Part model, mm, in its own coordinate system. Face numbers are marked on the shaded views. A direction names the side the tool comes from. Coordinates: 2 decimals unless noted, no trailing zeros. Order: outer loops, then holes, each group sorted by start corner. A loop starts at its lowest first (then second) coordinate and runs counter-clockwise, first axis right, second up.
from build123d import *

# Parameters (mm, degrees)
F0_W     = 25.2
F0_H     = 7.2
F1_DEPTH = 58.45
F2_W     = 15.086318
F2_H     = 7.2
F3_DEPTH = 5


with BuildPart() as f1:
    # F0 (on Front) → F1 (new body, symmetric)
    with BuildSketch(Plane.XZ):
        with Locations((-28.073686, 3.6)):
            Rectangle(F0_W, F0_H)
    extrude(amount=F1_DEPTH, both=True)

    # F2 (on face) → F3 (join)
    with BuildSketch(Plane.XZ.offset(58.45)):
        with Locations((-28.144586, 3.6)):
            Rectangle(F2_W, F2_H)
    extrude(amount=F3_DEPTH)


solid = f1.part
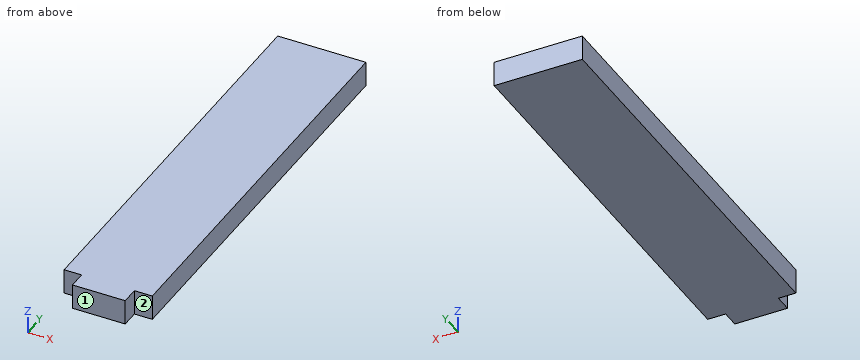
Q1. Pin check, flat tips, straight feed: pin 1 Ø4 at (x, z) = (-38, 4.5) entering from -Y; pin 2 Ø1 at (x, y) = (-29.5, 17.5) entering from -Z. Stop position of each tip, or through.
Results list:
pin 1: stops at y = -58.45
pin 2: stops at z = 0
Q2. Wall check: line 1 along Y through (x, z) = (-16.5, 1.75). Give the ranges that are in metal, low to high.
Results list:
line 1: y = -58.45 to 58.45
Q3. Cut at A-A on z = 5. Write the cut outline in (x, y).
Results list:
outline: (-40.67, -58.45) - (-35.69, -58.45) - (-35.69, -63.45) - (-20.6, -63.45) - (-20.6, -58.45) - (-15.47, -58.45) - (-15.47, 58.45) - (-40.67, 58.45) - close
Q4. Which spindle directions (+Z, -Z, +X, -X, +Y, -Y) get a long thin tool onto all of the face, cutting with end or side? Do the marked faces 1 and 2. Say none if no direction does.
Results list:
face 1: +Z, -Z, +X, -X, -Y
face 2: +Z, -Z, +X, -Y
Q5. Cut at B-B on x = -37. Write the cut outline in (y, z).
Results list:
outline: (-58.45, 0) - (58.45, 0) - (58.45, 7.2) - (-58.45, 7.2) - close
